Work out the finished part from the listing and answer in its coordinate system (mm). Face numbers are marked on the shaded views. A direction names the side the tool comes from. Coordinates: 2 decimals unless noted, no trailing zeros. Loops run counter-clockwise (first coordinate to the right, second up) from the corner with the lowest first, then second, coordinate; pieces in that order, holes last. Notation, with made-up numbers: (38, 2) -> (63, 2) arc R19 cw to (63, 31) -> close; hole circle Ø11 at (56, 12). An arc over 180 degrees is marked (long way). Use a Markdown table: item, result.
from build123d import *

# Parameters (mm, degrees)
F0_W     = 35
F0_H     = 35
F1_DEPTH = 4
F2_R     = 3
F2_R_2   = 1.675
F4_DEPTH = 2
F5_R     = 5
F6_DEPTH = 25
F3_W     = 35
F3_H     = 6
F7_DEPTH = 29
F9_DEPTH = 25


with BuildPart() as f1:
    # F0 (on Top) → F1 (new body)
    with BuildSketch(Plane.XY):
        with Locations((17.5, 17.5)):
            Rectangle(F0_W, F0_H)
    extrude(amount=F1_DEPTH)

    # F2 (on face) → F4 (cut)
    with BuildSketch(Plane.XY.offset(4)):
        with BuildLine():
            ThreePointArc((13, 21), (10, 24), (7, 21))
            ThreePointArc((7, 21), (10, 18), (13, 21))
        make_face()
        with BuildLine():
            ThreePointArc((8.325, 21), (10, 22.675), (11.675, 21))
            ThreePointArc((11.675, 21), (10, 19.325), (8.325, 21))
        make_face(mode=Mode.SUBTRACT)
        with Locations((25, 21)):
            Circle(F2_R)
        with Locations((25, 21)):
            Circle(F2_R_2, mode=Mode.SUBTRACT)
        with Locations((25, 6)):
            Circle(F2_R)
        with Locations((25, 6)):
            Circle(F2_R_2, mode=Mode.SUBTRACT)
        with BuildLine():
            ThreePointArc((13, 6), (7.87868, 8.12132), (10, 3))
            ThreePointArc((10, 3), (12.12132, 3.87868), (13, 6))
        make_face()
        with BuildLine():
            ThreePointArc((11.675, 6), (11.184404, 4.815596), (10, 4.325))
            ThreePointArc((10, 4.325), (8.815596, 7.184404), (11.675, 6))
        make_face(mode=Mode.SUBTRACT)
    extrude(amount=-F4_DEPTH, mode=Mode.SUBTRACT)

    # F5
    f5_edges = [f1.edges().sort_by_distance(p)[0] for p in [
        (0, 0, 2),
        (35, 0, 2),
    ]]
    fillet(f5_edges, radius=F5_R)

    # F2 (on face) → F6 (cut)
    with BuildSketch(Plane.XY.offset(4)):
        with BuildLine():
            ThreePointArc((8.325, 21), (10, 19.325), (11.675, 21))
            ThreePointArc((11.675, 21), (10, 22.675), (8.325, 21))
        make_face()
        with Locations((25, 21)):
            Circle(F2_R_2)
        with Locations((25, 6)):
            Circle(F2_R_2)
        with BuildLine():
            ThreePointArc((11.675, 6), (8.815596, 7.184404), (10, 4.325))
            ThreePointArc((10, 4.325), (11.184404, 4.815596), (11.675, 6))
        make_face()
    extrude(amount=-F6_DEPTH, mode=Mode.SUBTRACT)

    # F3 (on face) → F7 (join)
    with BuildSketch(Plane.XY.offset(4)):
        with Locations((17.5, 32)):
            Rectangle(F3_W, F3_H)
    extrude(amount=F7_DEPTH)

    # F8 (on face) → F9 (join)
    with BuildSketch(Plane.XZ.offset(-29)):
        Polygon((22.5, 33), (17.5, 33), (12.5, 33), (12.5, 29), (22.5, 29), align=None)
    extrude(amount=F9_DEPTH)


solid = f1.part
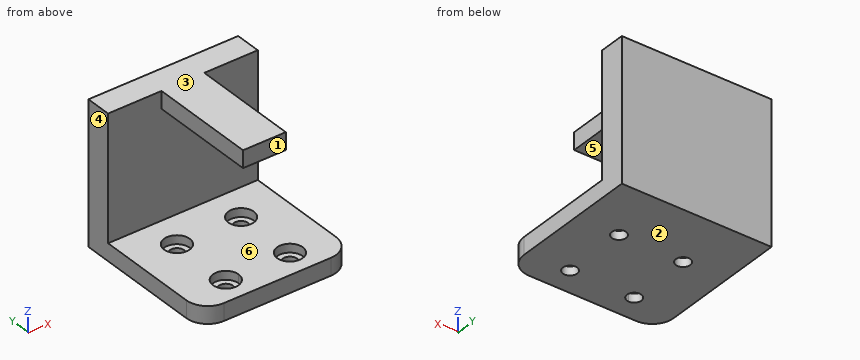
Q1. Section D-D on x = 13.5 is taken. Determine the outline of the cut face in (y, z), and give its area (3 significant figures).
Solved:
| item | result |
|---|---|
| outline | (0, 0) -> (35, 0) -> (35, 33) -> (4, 33) -> (4, 29) -> (29, 29) -> (29, 4) -> (0, 4) -> close |
| area | 414 mm² |
Q2. Section C-C on y = 21 is taken. Determine the outline of the cut face in (x, z) (3 decimals).
Solved:
| item | result |
|---|---|
| outline | (0, 0) -> (8.325, 0) -> (8.325, 2) -> (7, 2) -> (7, 4) -> (0, 4) -> close; (11.675, 0) -> (23.325, 0) -> (23.325, 2) -> (22, 2) -> (22, 4) -> (13, 4) -> (13, 2) -> (11.675, 2) -> close; (12.5, 29) -> (22.5, 29) -> (22.5, 33) -> (12.5, 33) -> close; (26.675, 0) -> (35, 0) -> (35, 4) -> (28, 4) -> (28, 2) -> (26.675, 2) -> close |
Q3. Given pin 1 Ø2 at (y, z) = (15.5, 31.5) entering from +X; pin 2 Ø1.2 at (x, z) = (18, 31.5) entering from -Y; pin 3 Ø3 at (x, y) = (10, 21.5) entering from +Z; pin 4 Ø2.5 at (x, y) = (10, 6) entering from -Z, each flat-ended and moving along its own axis, determine where each tip first touches the part or whether it passes through.
Solved:
| item | result |
|---|---|
| pin 1 | x = 22.5 |
| pin 2 | y = 4 |
| pin 3 | z = 2 |
| pin 4 | through |
Q4. For the marked faces 1 and 2, determine the directions among +Z, -Z, +X, -X, +Y, -Y from which every point of the face is accessible in a straight line to the end or side of a thin tool.
Solved:
| item | result |
|---|---|
| face 1 | +Z, +X, -X, -Y |
| face 2 | -Z, +X, -X, +Y, -Y |
Q5. Section B-B on x = 25 is taken. Determine the outline of the cut face in (y, z) (3 decimals).
Solved:
| item | result |
|---|---|
| outline | (0, 0) -> (4.325, 0) -> (4.325, 2) -> (3, 2) -> (3, 4) -> (0, 4) -> close; (7.675, 0) -> (19.325, 0) -> (19.325, 2) -> (18, 2) -> (18, 4) -> (9, 4) -> (9, 2) -> (7.675, 2) -> close; (22.675, 0) -> (35, 0) -> (35, 33) -> (29, 33) -> (29, 4) -> (24, 4) -> (24, 2) -> (22.675, 2) -> close |
Q6. Section A-A on y = 15 is taken. Determine the outline of the cut face in (x, z), and give its area (3 significant figures).
Solved:
| item | result |
|---|---|
| outline | (0, 0) -> (35, 0) -> (35, 4) -> (0, 4) -> close; (12.5, 29) -> (22.5, 29) -> (22.5, 33) -> (12.5, 33) -> close |
| area | 180 mm² |
Q7. Determine the mould class of the marked faces 3, 4, 5 and 6 for opening direction Z: pulls with the +Z half, pulls with the -Z half, needs draft (parallel to the pull), parting line crosses it, or undercut.
Solved:
| item | result |
|---|---|
| face 3 | pulls with the +Z half |
| face 4 | needs draft |
| face 5 | undercut |
| face 6 | undercut |
Q8. Consider line 1 (Y direction, x = 25, z = 3); line 2 (Y direction, x = 10, z = 1) (3 decimals); line 3 (Z direction, x = 18, y = 11). Determine where each line is inside the solid, lowest interval first. Write a range as [from, to].
Solved:
| item | result |
|---|---|
| line 1 | [0, 3], [9, 18], [24, 35] |
| line 2 | [0, 4.325], [7.675, 19.325], [22.675, 35] |
| line 3 | [0, 4], [29, 33] |
